Input: part model. Units: mm. Frame: model coordinates. Round coordinates to 2 decimals unless told otherwise and drop trailing zeros. Write each loop counter-clockwise with the first axis right and the second up, starting at its lowest first coordinate (ties: lowest second). Pieces come first, ordered by that corner, then holes. Notation, with made-up numbers: M -23.75,1 L 33.25,1 A13 ccw 33.25,19 Z; hole C 42,42.25 d10. An arc over 180 degrees is marked long. Write each question's results on one line, items separated by ' | '. Start each with the question number.
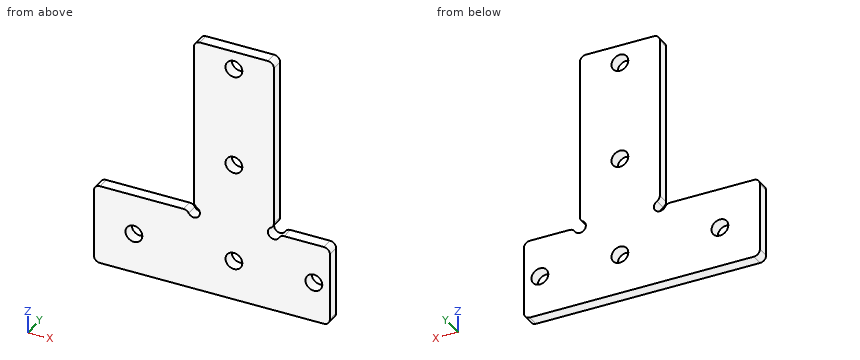
```python
from build123d import *

# Parameters (mm, degrees)
SKETCH_1_R          = 2.1
EXTRUDE_1_DEPTH     = 3
SKETCH_2_W          = 20
SKETCH_2_H          = 5.5
CUT_EXTRUDE_1_DEPTH = 3
SKETCH_3_R          = 1.5
CUT_EXTRUDE_3_DEPTH = 3
FILLET_2_R          = 1.5


with BuildPart() as part:
    # 草图1 → 凸台-拉伸1 (new body)
    with BuildSketch(Plane(origin=(0, 0, 0), x_dir=(1, 0, 0), z_dir=(0, 1, 0))):
        Polygon((-35, 10), (24, 10), (24, -10), (10, -10), (10, -60), (-10, -60), (-10, -10), (-35, -10), align=None)
        with Locations(Location((0, 0, 0), (0, 0, 270))):
            Circle(SKETCH_1_R, mode=Mode.SUBTRACT)
        with Locations(Location((20, 0, 0), (0, 0, 270))):
            Circle(SKETCH_1_R, mode=Mode.SUBTRACT)
        with Locations(Location((-25, 0, 0), (0, 0, 270))):
            Circle(SKETCH_1_R, mode=Mode.SUBTRACT)
        with Locations(Location((0, -25, 0), (0, 0, 270))):
            Circle(SKETCH_1_R, mode=Mode.SUBTRACT)
        with Locations(Location((0, -50, 0), (0, 0, 270))):
            Circle(SKETCH_1_R, mode=Mode.SUBTRACT)
    extrude(amount=EXTRUDE_1_DEPTH)

    # 草图2 → 切除-拉伸1 (cut)
    with BuildSketch(Plane(origin=(0, 3, 0), x_dir=(1, 0, 0), z_dir=(0, 1, 0))):
        with Locations((0, -57.25)):
            Rectangle(SKETCH_2_W, SKETCH_2_H)
    extrude(amount=-CUT_EXTRUDE_1_DEPTH, mode=Mode.SUBTRACT)

    # 草图3 → 切除-拉伸3 (cut)
    with BuildSketch(Plane(origin=(0, 3, 0), x_dir=(1, 0, 0), z_dir=(0, 1, 0))):
        with Locations((10, -10)):
            Circle(SKETCH_3_R)
        with Locations((-10, -10)):
            Circle(SKETCH_3_R)
    extrude(amount=-CUT_EXTRUDE_3_DEPTH, mode=Mode.SUBTRACT)

    # 圆角2
    fillet_2_edges = [part.edges().sort_by_distance(p)[0] for p in [
        (-35, 1.5, 10),
        (-35, 1.5, -10),
        (24, 1.5, -10),
        (24, 1.5, 10),
        (-10, 1.5, 54.5),
        (10, 1.5, 54.5),
        (11.5, 1.5, 10),
        (-10, 1.5, 11.5),
        (10, 1.5, 11.5),
        (-11.5, 1.5, 10),
    ]]
    fillet(fillet_2_edges, radius=FILLET_2_R)


solid = part.part
```
1. Contact query for flat-ended pins moving along their axis: P1, Ø6.5, axis at x = 0, z = 25, coming from the -Y side; P2, Ø0.9, axis at x = 19.5, y = 1.5, coming from the +Z side. Output: stop coordinate, or through.
2. Cut plane B-B on z = 25. Output: boundary loops of the cut face in (x, y).
3. Cut plane D-D on z = 0. Output: boundary loops of the cut face in (x, y).
4. Line query: L1, parallel to X at y = 2.45, z = 0; L2, parallel to X at y = 0.65, z = 0.5; L3, parallel to X at y = 2.45, z = 50. Output: solid intervals per line, ascending. Write a range as from..to.
5. Cut plane C-C on y = 0.75. Output: boundary loops of the cut face in (x, z).
6. Cut plane A-A on x = -25. Output: boundary loops of the cut face in (y, z), and give its area (3 significant figures).
Answers follow:
1) P1: stops at y = 0 | P2: stops at z = 10
2) outline: M -10,0 L -2.1,0 L -2.1,3 L -10,3 Z; M 2.1,0 L 10,0 L 10,3 L 2.1,3 Z
3) outline: M -35,0 L -27.1,0 L -27.1,3 L -35,3 Z; M -22.9,0 L -2.1,0 L -2.1,3 L -22.9,3 Z; M 2.1,0 L 17.9,0 L 17.9,3 L 2.1,3 Z; M 22.1,0 L 24,0 L 24,3 L 22.1,3 Z
4) L1: x = -35..-27.1, -22.9..-2.1, 2.1..17.9, 22.1..24 | L2: x = -35..-27.04, -22.96..-2.04, 2.04..17.96, 22.04..24 | L3: x = -10..-2.1, 2.1..10
5) outline: M -35,-8.5 A1.5 ccw -33.5,-10 L 22.5,-10 A1.5 ccw 24,-8.5 L 24,8.5 A1.5 ccw 22.5,10 L 12.6,10 A1.5 ccw 11.3,9.25 A1.5 cw long 9.25,11.3 A1.5 ccw 10,12.6 L 10,53 A1.5 ccw 8.5,54.5 L -8.5,54.5 A1.5 ccw -10,53 L -10,12.6 A1.5 ccw -9.25,11.3 A1.5 cw long -11.3,9.25 A1.5 ccw -12.6,10 L -33.5,10 A1.5 ccw -35,8.5 Z; hole C -25,0 d4.2; hole C 0,0 d4.2; hole C 0,25 d4.2; hole C 0,50 d4.2; hole C 20,0 d4.2
6) outline: M 0,-10 L 3,-10 L 3,-2.1 L 0,-2.1 Z; M 0,2.1 L 3,2.1 L 3,10 L 0,10 Z | area: 47.4 mm2
